Autodesk Inventor part; units mm, degrees
ref_plane "YZ Plane" through (0, 0, 0) normal (1, 0, 0) x (0, 1, 0)
ref_plane "XZ Plane" through (0, 0, 0) normal (0, 1, 0) x (-1, 0, 0)
ref_plane "XY Plane" through (0, 0, 0) normal (0, 0, 1) x (1, 0, 0)
sketch "Sketch1" plane through (0, 0, 0) normal (0, 1, 0) x (-1, 0, 0)
  line L0 (50.7746, 6.35) -> (47.625, 6.35)
  line L1 (47.625, 6.35) -> (47.625, -6.35)
  line L2 (47.625, -6.35) -> (50.7746, -6.35)
  line L3 (50.7746, -6.35) -> (50.7746, 6.35)
  arc A0 (47.625, -2.9696) -> (47.625, 2.9696) centre (45.9105, 0) ccw
  line L4 (0, -8.89) -> (0, 8.89)
  point P0 (0, 0)
  point P1 (50.7746, 0)
  dimension "d1" = 47.625
  dimension "d2" = 3.1496
  dimension "d3" = 6.35
  dimension "d4" = 6.35
  dimension "d5" = 1.7145
  dimension "d6" = 3.429
revolve "Revolution1" add sketch "Sketch1" angle 360 about axis through (0, 0, -10) along (0, 0, 1) contours L3 L2 L1 A0 L0
sketch "Sketch2" plane through (0, 0, -6.35) normal (0, 0, -1) x (-1, 0, 0)
  circle A0 centre (0, 0) radius 50.7746
  circle A1 centre (0, 0) radius 47.625
  circle A2 centre (0, 0) radius 53.9496
  dimension "d8" = 3.175
extrude "Extrusion1" add sketch "Sketch2" along normal blind 6.35 contours A0
sketch "Sketch3" plane through (0, 0, -12.7) normal (0, 0, -1) x (-1, 0, 0)
  circle A0 centre (0, 0) radius 53.9496
  circle A1 centre (0, 0) radius 47.625
extrude "Extrusion2" add sketch "Sketch3" along normal blind 3.175
properties part number "outer ring end stop"
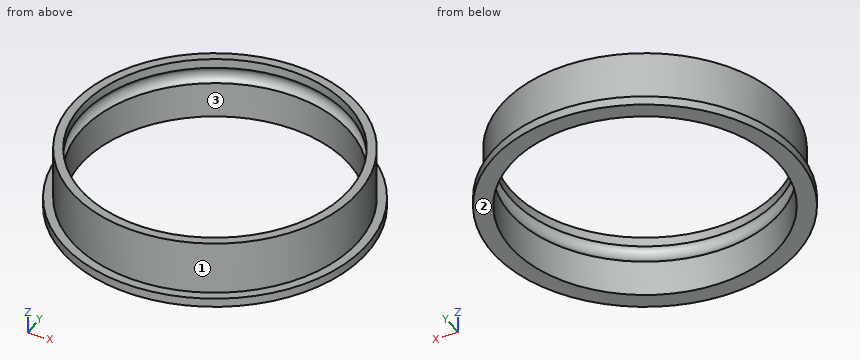
Build history of the part. All positions in model axes, mm. Face numbers are marked on the shaded views. Round coordinates to 2 decimals unless told otherwise and drop trailing zeros. Loops run counter-clockwise (first coordinate to the right, second up) from the corner with the lowest first, then second, coordinate; pieces in that order, holes last.
Item 1: Saw through at C-C (z = -10.75). List the corners of the cut face in (x, y) (3 decimals).
Item 2: Two-plate mould, pull along X, no slides. Class the marked faces 1, 2 and 3: released by +X, released by -X, zero draft, split by the parting line, or undercut.
Item 3: Drill centre lines: line 1 along Y through (x, z) = (0, 5.3) (3 decimals); line 2 along X through (y, z) = (1, -9); line 3 along X through (y, z) = (-5.5, 4.5). Where is each one in solid material? Low to high.
Item 4: Pin check, flat tips, straight feed: P1, Ø5, axis at x = 12, z = 2, coming from the -Y side; P2, Ø1, axis at x = -5, z = 1, coming from the +Y side; P3, Ø2, axis at y = -18, z = -2, coming from the -X side. Stop position of each tip, or through.
Worked answers:
1. outline: circle Ø101.549 at (0, 0); hole circle Ø95.25 at (0, 0)
2. face 1: split by the parting line
2. face 2: zero draft
2. face 3: undercut
3. line 1: y = -50.775 to -47.625, 47.625 to 50.775
3. line 2: x = -50.76 to -47.61, 47.61 to 50.76
3. line 3: x = -50.48 to -47.31, 47.31 to 50.48
4. P1: stops at y = -49.88
4. P2: stops at y = 50.57
4. P3: stops at x = -47.84
